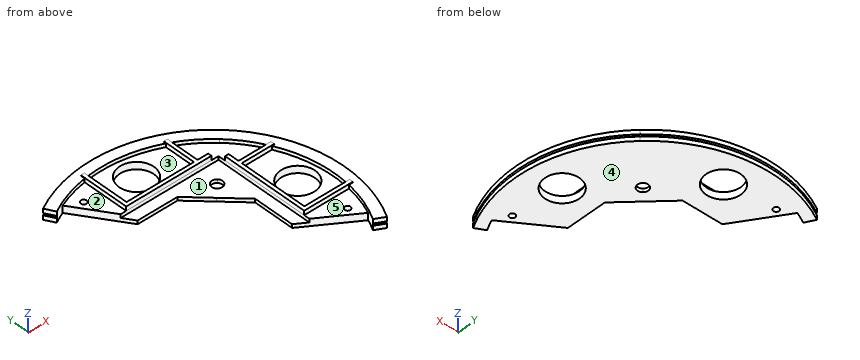
```python
from build123d import *

# Parameters (mm, degrees)
SKETCH004_W                    = 42
SKETCH004_H                    = 42
PAD001_DEPTH                   = 1
SKETCH003_R                    = 4.8856059565
SKETCH003_R_2                  = 0.8
PAD_DEPTH                      = 2
PAD002_DEPTH                   = 1.2
SKETCH008_W                    = 3
SKETCH008_H                    = 0.6
POCKET_DEPTH                   = 0.56
PART_MIRRORING_PLACEMENT_ANGLE = 90.0000000001


with BuildPart() as sweep_body:
    # Sweep: sweep along a path in Sketch002
    with BuildLine(Plane.XY) as sweep_path:
        ThreePointArc((30.6116897499, -16.9683367086), (34.659382406, 4.8710585336), (24.7487373415, 24.7487373415))
    # Sketch → Sweep (sweep)
    with BuildSketch(Plane(origin=(0, 0, -2), x_dir=(1, 0, 0), z_dir=(0, -1, 0))):
        Polygon((34, 3), (37, 3), (37, 1.8), (36.7, 1.5), (37, 1.2), (37, 0), (34, 0), align=None)
    sweep(path=sweep_path.line)


with BuildPart() as pad001:
    # Sketch004 → Pad001 (new body)
    with BuildSketch(Plane.XY):
        Rectangle(SKETCH004_W, SKETCH004_H)
    extrude(amount=-PAD001_DEPTH)


with BuildPart() as pocket:
    # Sketch003 → Pad (new body)
    with BuildSketch(Plane.XY):
        with BuildLine():
            ThreePointArc((32.0633897526, -14.0334969831), (34.3936021818, 6.4869198359), (24.7487373415, 24.7487373415))
            Line((24.7487373415, 24.7487373415), (16.5606601718, 16.5606601718))
            ThreePointArc((14.4393398282, 14.4393398282), (16.5606601718, 14.4393398282), (16.5606601718, 16.5606601718))
            Line((14.4393398282, 14.4393398282), (12.3180194847, 12.3180194847))
            Line((18, 6.6360389693), (12.3180194847, 12.3180194847))
            Line((18, -4.584534), (18, 6.6360389693))
            Line((32.0633897526, -14.0334969831), (18, -4.584534))
        make_face()
        with Locations((27.575581, 4)):
            Circle(SKETCH003_R, mode=Mode.SUBTRACT)
        with Locations((29.091162, -9.5051)):
            Circle(SKETCH003_R_2, mode=Mode.SUBTRACT)
    extrude(amount=-PAD_DEPTH)

    # Cut: cut Pad001
    add(pad001.part, mode=Mode.SUBTRACT)

    # Fusion: union Sweep body
    add(sweep_body.part)

    # Sketch007 → Pad002 (new body)
    with BuildSketch(Plane.XY):
        Polygon((20.99856, 18.998371), (22, 18.998371), (22, 16), (31.146767, 16), (31.146767, 14.999727), (22, 14.999727), (22, -4), (34.761593, -4), (34.761593, -5.021452), (20.99856, -5.021452), align=None)
    extrude(amount=PAD002_DEPTH)

    # Sketch008 → Pocket (cut)
    with BuildSketch(Plane(origin=(0, 0, 0), x_dir=(0.8746197071, -0.4848096202, 0), z_dir=(-0.4848096202, -0.8746197071, 0))):
        with Locations((35.5, -0.5)):
            Rectangle(SKETCH008_W, SKETCH008_H)
    extrude(amount=-POCKET_DEPTH, mode=Mode.SUBTRACT)


with BuildPart() as fusion001:
    # Part__Mirroring: instance of Pocket
    add(pocket.part.mirror(Plane(origin=(0, 0, 0), x_dir=(1, 0, 0), z_dir=(0, 1, 0))))


with BuildPart() as fusion001_1:
    # Part__Mirroring placement: moved
    add(fusion001.part.rotate(Axis((0, 0, 0), (0, 0, 1)), PART_MIRRORING_PLACEMENT_ANGLE))

    # Fusion001: union Pocket
    add(pocket.part)


solid = fusion001_1.part
```
For this review, take the finished solid that the model builds, in its own axes (mm). Face numbers are marked on the shaded views. A direction names the side the tool comes from. Coordinates: 2 decimals unless noted, no trailing zeros. Answer as a JSON object with one key per item and string values. Group by question number.
1. For probe 1 along Y at (x, z) = (23, 0.3); probe 2 along X at (y, z) = (28.5, -0.7); probe 3 along Y at (x, z) = (26.5, -1.4), list the stretches that pass through material, from the lowest coordinate up.
2. For the marked faces 1, 2 and 3, list the 3-axis set-ups (+Z, -Z, +X, -X, +Y, -Y) from which the entire face can be reached by the end or side of a thin tool; tool diameter is ignored.
3. The part is to be moulded in two halves that separate along Y. For the marked faces 4 and 5, say which applies: pulls with the +Y half, pulls with the -Y half, needs draft (parallel to the pull), parting line crosses it, or undercut.
4. Clearance check with flat-ended pins moving along their axes: P1, Ø1, axis at y = -11, z = -1, coming from the -X side; P2, Ø1.3, axis at x = 27.5, z = 1, coming from the -Y side; P3, Ø6, axis at x = 29, y = 8.5, coming from the +Z side. State where each tip first meets the part, or that it passes through.
Final values:
{
 "1": {"probe 1": "-5.02 to -4, 15 to 16, 25.04 to 28.98", "probe 2": "-11.64 to -10.04, -8.97 to -0.8, 8.8 to 23.44", "probe 3": "-10.3 to -0.77, 8.77 to 25.82"},
 "2": {"face 1": "+Z, -X, -Y", "face 2": "+Z, -Y", "face 3": "+Z"},
 "3": {"face 4": "needs draft", "face 5": "undercut"},
 "4": {"P1": "x = 26.8", "P2": "y = -5.02", "P3": "z = 0"}
}
